For this review, take the finished solid that the model builds, in its own axes (mm). A direction names the side the tool comes from. Round coordinates to 2 decimals unless told otherwise and drop trailing zeros. Loops run counter-clockwise (first coordinate to the right, second up) from the corner with the lowest first, then second, coordinate; pieces in that order, holes last.
1) Tool access review of faces 4 (the cylindrical face through (19, 75, 0)), 5 (the flat face through (0, 149, -13)), 6 (the cylindrical face through (-21.494, 66.204, -0.286)), 7 (the flat face through (0, 149, -15)): name each direction out of +Z, -Z, +X, -X, +Y, -Y from which nothing blocks a thin tool from reaching the whole face with its end or side.
2) Insertion check: pin 1 (5 mm diameter, centred on x = -26.6, z = -11.6, fed in from -Y); pin 2 (8 mm diameter, centred on y = 185, z = -3.5, fed in from -X); pin 3 (1.3 mm diameter, centred on y = 152.5, z = 6, fed in from +X). Each pin has a flat end and moves straight along its axis. Give the tip position at first contact, or say it passes through.
3) Wall thickness on L1, parallel to X at y = 185.5, z = 0; L2, parallel to X at y = 117, z = -11.6; L3, parallel to Z at x = -27, y = 204: over which ranges is each line inside the solid? List them lowest first.
4) Take a section at B-B (y = 91). Give the number of separate pieces and of enclosed holes in the cut face, then the cut area to 3 significant figures.
5) Mouldability with a two-part tool opening along Y and no side actions: class faces 1 (the flat face through (2, 70, 0)), 2 (the flat face through (7.378, 149.006, -6.208)), 3 (the flat face through (-18, 70, 3)) as pulls with the +Y half, pulls with the -Y half, needs draft (parallel to the pull), parting line crosses it, or undercut.
6) Take a section at A-A (x = 100). State the section outline as (y, z) points, then the cut area to 3 significant figures.
7) Take a section at C-C (x = -77). State the section outline as (y, z) points, then the cut area to 3 significant figures.
```python
from build123d import *

# Parameters (mm, degrees)
SKETCH1_W                = 32
SKETCH1_H                = 9
BOSS_EXTRUDE1_DEPTH      = 125
TAP1_D                   = 10.106
SKETCH4_R                = 4.5
CUT_EXTRUDE1_DEPTH       = 127.340808926
SKETCH5_R                = 2.1
SKETCH5_R_2              = 3.3235
BOSS_EXTRUDE2_DEPTH      = 142
CUT_EXTRUDE2_DEPTH       = 4
CHAMFER1_SIZE            = 0.3
CHAMFER1_OF_MIRROR1_SIZE = 0.3


with BuildPart() as part:
    # Sketch1 → Boss-Extrude1 (new, symmetric)
    with BuildSketch(Plane(origin=(0, 0, 0), x_dir=(0, 0, -1), z_dir=(1, 0, 0))):
        with Locations((0, 74.5)):
            Rectangle(SKETCH1_W, SKETCH1_H)
    extrude(amount=BOSS_EXTRUDE1_DEPTH, both=True)

    # Tap1 (through all)
    with Locations(Plane(origin=(0, 79, 0), x_dir=(1, 0, 0), z_dir=(0, 1, 0))):
        with Locations((-100, 0), (100, 0)):
            Hole(TAP1_D / 2)

    # Sketch4 → Cut-Extrude1 (cut, through all)
    with BuildSketch(Plane(origin=(0, 79, 0), x_dir=(1, 0, 0), z_dir=(0, 1, 0))):
        with Locations(Location((-15, 0, 0), (0, 0, 270))):
            Circle(SKETCH4_R)
        with Locations(Location((15, 0, 0), (0, 0, 270))):
            Circle(SKETCH4_R)
    extrude(amount=-CUT_EXTRUDE1_DEPTH, mode=Mode.SUBTRACT)

    # Sketch5 → Boss-Extrude2 (add)
    with BuildSketch(Plane(origin=(0, 79, 0), x_dir=(1, 0, 0), z_dir=(0, 1, 0))):
        with BuildLine():
            Line((-11, -15), (11, -15))
            Line((11, -15), (11, -13))
            Line((11, -13), (6.75, -13))
            Line((6.75, -13), (6.75, -9.664213562))
            Line((6.75, -9.664213562), (10.414213562, -6))
            Line((10.414213562, -6), (14.480384758, -6))
            Line((14.480384758, -6), (15, -5.7))
            Line((15, -5.7), (15.519615242, -6))
            Line((15.519615242, -6), (19.585786438, -6))
            Line((19.585786438, -6), (23.25, -9.664213562))
            Line((23.25, -9.664213562), (23.25, -13))
            Line((23.25, -13), (19, -13))
            Line((19, -13), (19, -15))
            Line((19, -15), (28, -15))
            ThreePointArc((28, -15), (29.414213562, -14.414213562), (30, -13))
            Line((30, -13), (30, -4))
            Line((30, -4), (28, -4))
            Line((28, -4), (28, -8.25))
            Line((28, -8.25), (24.664213562, -8.25))
            Line((24.664213562, -8.25), (21, -4.585786438))
            Line((21, -4.585786438), (21, -0.519615242))
            Line((21, -0.519615242), (20.7, 0))
            Line((20.7, 0), (21, 0.519615242))
            Line((21, 0.519615242), (21, 4.585786438))
            Line((21, 4.585786438), (24.664213562, 8.25))
            Line((24.664213562, 8.25), (28, 8.25))
            Line((28, 8.25), (28, 4))
            Line((28, 4), (30, 4))
            Line((30, 4), (30, 13))
            ThreePointArc((30, 13), (29.414213562, 14.414213562), (28, 15))
            Line((28, 15), (19, 15))
            Line((19, 15), (19, 13))
            Line((19, 13), (23.25, 13))
            Line((23.25, 13), (23.25, 9.664213562))
            Line((23.25, 9.664213562), (19.585786438, 6))
            Line((19.585786438, 6), (15.519615242, 6))
            Line((15.519615242, 6), (15, 5.7))
            Line((15, 5.7), (14.480384758, 6))
            Line((14.480384758, 6), (10.414213562, 6))
            Line((10.414213562, 6), (6.75, 9.664213562))
            Line((6.75, 9.664213562), (6.75, 13))
            Line((6.75, 13), (11, 13))
            Line((11, 13), (11, 15))
            Line((11, 15), (-11, 15))
            Line((-11, 15), (-11, 13))
            Line((-11, 13), (-6.75, 13))
            Line((-6.75, 13), (-6.75, 9.664213562))
            Line((-6.75, 9.664213562), (-10.414213562, 6))
            Line((-10.414213562, 6), (-14.480384758, 6))
            Line((-14.480384758, 6), (-15, 5.7))
            Line((-15, 5.7), (-15.519615242, 6))
            Line((-15.519615242, 6), (-19.585786438, 6))
            Line((-19.585786438, 6), (-23.25, 9.664213562))
            Line((-23.25, 9.664213562), (-23.25, 13))
            Line((-23.25, 13), (-19, 13))
            Line((-19, 13), (-19, 15))
            Line((-19, 15), (-28, 15))
            ThreePointArc((-28, 15), (-29.414213562, 14.414213562), (-30, 13))
            Line((-30, 13), (-30, 4))
            Line((-30, 4), (-28, 4))
            Line((-28, 4), (-28, 8.25))
            Line((-28, 8.25), (-24.664213562, 8.25))
            Line((-24.664213562, 8.25), (-21, 4.585786438))
            Line((-21, 4.585786438), (-21, 0.519615242))
            Line((-21, 0.519615242), (-20.7, 0))
            Line((-20.7, 0), (-21, -0.519615242))
            Line((-21, -0.519615242), (-21, -4.585786438))
            Line((-21, -4.585786438), (-24.664213562, -8.25))
            Line((-24.664213562, -8.25), (-28, -8.25))
            Line((-28, -8.25), (-28, -4))
            Line((-28, -4), (-30, -4))
            Line((-30, -4), (-30, -13))
            ThreePointArc((-30, -13), (-29.414213562, -14.414213562), (-28, -15))
            Line((-28, -15), (-19, -15))
            Line((-19, -15), (-19, -13))
            Line((-19, -13), (-23.25, -13))
            Line((-23.25, -13), (-23.25, -9.664213562))
            Line((-23.25, -9.664213562), (-19.585786438, -6))
            Line((-19.585786438, -6), (-15.519615242, -6))
            Line((-15.519615242, -6), (-15, -5.7))
            Line((-15, -5.7), (-14.480384758, -6))
            Line((-14.480384758, -6), (-10.414213562, -6))
            Line((-10.414213562, -6), (-6.75, -9.664213562))
            Line((-6.75, -9.664213562), (-6.75, -13))
            Line((-6.75, -13), (-11, -13))
            Line((-11, -13), (-11, -15))
        make_face()
        with Locations(Location((-26.6, -11.6, 0), (0, 0, 270))):
            Circle(SKETCH5_R, mode=Mode.SUBTRACT)
        with Locations(Location((-26.6, 11.6, 0), (0, 0, 270))):
            Circle(SKETCH5_R, mode=Mode.SUBTRACT)
        with Locations(Location((-15, 0, 0), (0, 0, 270))):
            Circle(SKETCH5_R_2, mode=Mode.SUBTRACT)
        with Locations(Location((26.6, -11.6, 0), (0, 0, 270))):
            Circle(SKETCH5_R, mode=Mode.SUBTRACT)
        with Locations(Location((15, 0, 0), (0, 0, 270))):
            Circle(SKETCH5_R_2, mode=Mode.SUBTRACT)
        with Locations(Location((26.6, 11.6, 0), (0, 0, 270))):
            Circle(SKETCH5_R, mode=Mode.SUBTRACT)
        with BuildLine():
            Line((4.75, 8.835786438), (4.75, 12))
            ThreePointArc((4.75, 12), (4.457106781, 12.707106781), (3.75, 13))
            Line((3.75, 13), (-3.75, 13))
            ThreePointArc((-3.75, 13), (-4.457106781, 12.707106781), (-4.75, 12))
            Line((-4.75, 12), (-4.75, 8.835786438))
            Line((-4.75, 8.835786438), (-9.933994275, 3.651792162))
            ThreePointArc((-9.933994275, 3.651792162), (-10.020243756, 3.470780401), (-9.973202134, 3.275866789))
            ThreePointArc((-9.973202134, 3.275866789), (-9, 0), (-9.973202134, -3.275866789))
            ThreePointArc((-9.973202134, -3.275866789), (-10.020243756, -3.470780401), (-9.933994275, -3.651792162))
            Line((-9.933994275, -3.651792162), (-4.75, -8.835786438))
            Line((-4.75, -8.835786438), (-4.75, -12))
            ThreePointArc((-4.75, -12), (-4.457106781, -12.707106781), (-3.75, -13))
            Line((-3.75, -13), (3.75, -13))
            ThreePointArc((3.75, -13), (4.457106781, -12.707106781), (4.75, -12))
            Line((4.75, -12), (4.75, -8.835786438))
            Line((4.75, -8.835786438), (9.933994275, -3.651792162))
            ThreePointArc((9.933994275, -3.651792162), (10.020243756, -3.470780401), (9.973202134, -3.275866789))
            ThreePointArc((9.973202134, -3.275866789), (9, 0), (9.973202134, 3.275866789))
            ThreePointArc((9.973202134, 3.275866789), (10.020243756, 3.470780401), (9.933994275, 3.651792162))
            Line((9.933994275, 3.651792162), (4.75, 8.835786438))
        make_face(mode=Mode.SUBTRACT)
    extrude(amount=BOSS_EXTRUDE2_DEPTH)

    # Sketch6 → Revolve1 (revolve)
    with BuildSketch(Plane.XY, mode=Mode.PRIVATE) as revolve1_sk:
        Polygon((18, 62), (21.5, 62), (21.5, 70), (19, 70), (19, 95), (15, 95), (15, 67.732050808), (18, 66), align=None)
    revolve1 = revolve(revolve1_sk.sketch.rotate(Axis((15, 95, 0), (0, -1, 0)), 180), axis=Axis((15, 95, 0), (0, -1, 0)))

    # Sketch7 → Cut-Extrude2 (cut)
    with BuildSketch(Plane.XZ.offset(-62)):
        Polygon((18.464101615, 0), (16.732050808, 3), (13.267949192, 3), (11.535898385, 0), (13.267949192, -3), (16.732050808, -3), align=None)
    cut_extrude2 = extrude(amount=-CUT_EXTRUDE2_DEPTH, mode=Mode.SUBTRACT)

    # Chamfer1
    chamfer1_edges = [part.edges().sort_by_distance(p)[0] for p in [
        (21.5, 62, 0),
    ]]
    chamfer(chamfer1_edges, length=CHAMFER1_SIZE)

    # Mirror1: Revolve1, Cut-Extrude2 across plane
    add(revolve1.mirror(Plane(origin=(0, 0, 0), x_dir=(0, 0, 1), z_dir=(1, 0, 0))))
    add(cut_extrude2.mirror(Plane(origin=(0, 0, 0), x_dir=(0, 0, 1), z_dir=(1, 0, 0))), mode=Mode.SUBTRACT)

    # Chamfer1 of Mirror1
    chamfer1_of_mirror1_edges = [part.edges().sort_by_distance(p)[0] for p in [
        (-21.5, 62, 0),
    ]]
    chamfer(chamfer1_of_mirror1_edges, length=CHAMFER1_OF_MIRROR1_SIZE)


solid = part.part
```
Response:
1. face 4: none
1. face 5: +Y
1. face 6: -Y
1. face 7: -Z, +X, -X, +Y
2. pin 1: stops at y = 70
2. pin 2: stops at x = -30
2. pin 3: stops at x = 30
3. L1: x = -20.7 to -18.32, -11.68 to -9, 9 to 11.68, 18.32 to 20.7
3. L2: x = -30 to -28.7, -24.5 to -23.25, -6.75 to -4.75, 4.75 to 6.75, 23.25 to 24.5, 28.7 to 30
3. L3: z = -15 to -13.66, -9.54 to -8.25, 8.25 to 9.54, 13.66 to 15
4. separate pieces: 1
4. enclosed holes: 5
4. area: 664 mm2
5. face 1: pulls with the -Y half
5. face 2: needs draft
5. face 3: undercut
6. outline: (70, -16) - (79, -16) - (79, -5.05) - (70, -5.05) - close; (70, 5.05) - (79, 5.05) - (79, 16) - (70, 16) - close
6. area: 197 mm2
7. outline: (70, -16) - (79, -16) - (79, 16) - (70, 16) - close
7. area: 288 mm2
